from build123d import *

# Parameters (mm, degrees)
SKETCH1_W           = 935
SKETCH1_H           = 680
BOSS_EXTRUDE1_DEPTH = 210
BOSS_EXTRUDE2_DEPTH = 935
FILLET1_R           = 80


with BuildPart() as part:
    # Sketch1 → Boss-Extrude1 (new body)
    with BuildSketch(Plane(origin=(0, 0, 0), x_dir=(1, 0, 0), z_dir=(0, 1, 0))):
        with Locations((0, 340)):
            Rectangle(SKETCH1_W, SKETCH1_H)
    extrude(amount=-BOSS_EXTRUDE1_DEPTH)

    # Sketch3 → Boss-Extrude2 (add)
    with BuildSketch(Plane.ZY.offset(467.5)):
        Polygon((-70, 0), (-70, 50), (-430, 50), (-480, 0), align=None)
    extrude(amount=-BOSS_EXTRUDE2_DEPTH)

    # Fillet1
    # the kernel refuses this fillet: 80 mm, written as the material it takes off along each edge
    with BuildSketch(Plane(origin=(-652.904962177, 50, -70), x_dir=(0, -1, 0), z_dir=(1, 0, 0))) as fillet1_piece_1:
        with BuildLine():
            CenterArc((80, 74.161984871), FILLET1_R, 180, 67.975687163)
            Line((0, 74.161984871), (-1.6, 74.161984871))
            Line((-1.6, 74.161984871), (-1.6, 0))
            Line((-1.6, 0), (0, -1.6))
            ThreePointArc((0, -1.6), (25, -1.6), (49.4, -1.483239697))
            Line((49.4, -1.483239697), (50, 0))
        make_face()
    extrude(amount=1305.809924355, mode=Mode.SUBTRACT)
    with BuildSketch(Plane(origin=(-550.342712475, 50, -430), x_dir=(0, -0.7071067811865477, -0.7071067811865474), z_dir=(1, 0, 0))) as fillet1_piece_2:
        with BuildLine():
            CenterArc((FILLET1_R * 0.414213562373, -FILLET1_R), FILLET1_R, 90, 45)
            Line((-FILLET1_R * 0.292893218813, -FILLET1_R * 0.292893218813), (-FILLET1_R * 0.307035354437, -FILLET1_R * 0.27875108319))
            Line((-FILLET1_R * 0.307035354437, -FILLET1_R * 0.27875108319), (-FILLET1_R * 0.00828427124746, FILLET1_R * 0.02))
            Line((-FILLET1_R * 0.00828427124746, FILLET1_R * 0.02), (FILLET1_R * 0.414213562373, FILLET1_R * 0.02))
            Line((FILLET1_R * 0.414213562373, FILLET1_R * 0.02), (FILLET1_R * 0.414213562373, 0))
        make_face()
    extrude(amount=1100.685424949, mode=Mode.SUBTRACT)


solid = part.part
Could you check a few things on this model? Use its own coordinates, in mm. A direction names the side the tool comes from. Give positions to 0.01 mm unless a question says otherwise; leave off trailing zeros. Write each loop counter-clockwise with the first axis right and the second up, starting at its lowest first coordinate (ties: lowest second). Pieces come first, ordered by that corner, then holes. Notation, with made-up numbers: (85.5, 27) - (139.5, 27) arc R28 ccw to (139.5, 53) - close; hole circle Ø5 at (-35.75, 54.25). An arc over 180 degrees is marked (long way). Use CSV: the item, a comma, the result in double quotes. Start each with the question number.
Item 1: I want a section at B-B, the plane z = -510.5. Please give me the cut outline in (x, y), then the cut area to 3 significant figures.
Item 2: I want a section at A-A, the plane x = 142.5. Please give me the cut outline in (y, z).
Item 3: If we mould it in two halves opening along X, with no side actions, what happens to faces 3 (the face through (-7, 0, -581)), 4 (the face through (467.5, -78, -335)), 5 (the face through (-467.5, -78, -335))? For each: pulls with the +X half, pulls with the -X half, needs draft (parallel to the pull), parting line crosses it, or undercut.
Item 4: I want a section at C-C, the plane z = -108. Please give me the cut outline in (x, y).
Item 5: For faces 1 (the face through (-7, 0, -35)), 2 (the face through (-6.545, 43.741, -427.883)), which set-ups out of +Z, -Z, +X, -X, +Y, -Y let a thin tool reach every point of the face, with its end or its side?
Item 6: If I drill on line 1 along Y through (x, z) = (324.5, -56); line 2 along Y through (x, z) = (260, -434); line 3 along Z through (x, y) = (84, 23.5), over which ranges is the centre line in solid material (lowest first)?
Item 7: I'm going to push flat-ended pins straight in: pin 1 (8 mm diameter, centred on x = -310, y = 9.5, fed in from -Z); pin 2 (12 mm diameter, centred on x = -83.5, z = -599, fed in from +Y). Where does each tip first touch, or does it pass through?
Findings:
1,outline,"(-467.5, -210) - (467.5, -210) - (467.5, 0) - (-467.5, 0) - close"
1,area,"196,000 mm2"
2,outline,"(-210, -680) - (0, -680) - (0, -480) - (26.57, -453.43) arc R80 ccw to (50, -396.86) - (50, -144.16) arc R80 ccw to (0, -70) - (0, 0) - (-210, 0) - close"
3,face 3,"needs draft"
3,face 4,"pulls with the +X half"
3,face 5,"pulls with the -X half"
4,outline,"(-467.5, -210) - (467.5, -210) - (467.5, 41.36) - (-467.5, 41.36) - close"
5,face 1,"+Z, +X, -X, +Y"
5,face 2,"-Z, +X, -X, +Y"
6,line 1,"y = -210 to 0"
6,line 2,"y = -210 to 40.86"
6,line 3,"z = -456.5 to -84.68"
7,pin 1,"stops at z = -474.5"
7,pin 2,"stops at y = 0"
